from build123d import *

# Parameters (mm, degrees)
SKETCH1_W           = 261.5
SKETCH1_H           = 125.5
SKETCH1_R           = 2.5
SKETCH1_R_2         = 1.59
SKETCH1_R_3         = 2.1
SKETCH1_R_4         = 11.75
SKETCH1_W_2         = 33
SKETCH1_H_2         = 90
BOSS_EXTRUDE1_DEPTH = 5
CUT_EXTRUDE1_DEPTH  = 10
FILLET1_R           = 10
FILLET2_R           = 10


with BuildPart() as part:
    # Sketch1 → Boss-Extrude1 (new body)
    with BuildSketch(Plane.XY):
        with Locations((130.75, -62.75)):
            Rectangle(SKETCH1_W, SKETCH1_H)
        with Locations((255, -37.25)):
            Circle(SKETCH1_R, mode=Mode.SUBTRACT)
        with Locations((255, -88.25)):
            Circle(SKETCH1_R, mode=Mode.SUBTRACT)
        with Locations((183.81, -47.125)):
            Circle(SKETCH1_R_2, mode=Mode.SUBTRACT)
        with Locations((164.76, -78.375)):
            Circle(SKETCH1_R_2, mode=Mode.SUBTRACT)
        with Locations((152.06, -78.375)):
            Circle(SKETCH1_R_2, mode=Mode.SUBTRACT)
        with Locations((43.875030639, -118.888854871)):
            Circle(SKETCH1_R_3, mode=Mode.SUBTRACT)
        with Locations((183.81, -78.375)):
            Circle(SKETCH1_R_2, mode=Mode.SUBTRACT)
        with Locations((145.71, -47.125)):
            Circle(SKETCH1_R_2, mode=Mode.SUBTRACT)
        with Locations((158.41, -47.125)):
            Circle(SKETCH1_R_2, mode=Mode.SUBTRACT)
        with Locations((171.11, -47.125)):
            Circle(SKETCH1_R_2, mode=Mode.SUBTRACT)
        with Locations((145.71, -78.375)):
            Circle(SKETCH1_R_2, mode=Mode.SUBTRACT)
        with Locations((158.41, -78.375)):
            Circle(SKETCH1_R_2, mode=Mode.SUBTRACT)
        with Locations((171.11, -78.375)):
            Circle(SKETCH1_R_2, mode=Mode.SUBTRACT)
        with Locations((84.04, -78.375)):
            Circle(SKETCH1_R_2, mode=Mode.SUBTRACT)
        with Locations((96.74, -78.375)):
            Circle(SKETCH1_R_2, mode=Mode.SUBTRACT)
        with Locations((109.44, -78.375)):
            Circle(SKETCH1_R_2, mode=Mode.SUBTRACT)
        with Locations((84.04, -47.125)):
            Circle(SKETCH1_R_2, mode=Mode.SUBTRACT)
        with Locations((96.74, -47.125)):
            Circle(SKETCH1_R_2, mode=Mode.SUBTRACT)
        with Locations((109.44, -47.125)):
            Circle(SKETCH1_R_2, mode=Mode.SUBTRACT)
        with Locations((90.39, -78.375)):
            Circle(SKETCH1_R_2, mode=Mode.SUBTRACT)
        with Locations((103.09, -78.375)):
            Circle(SKETCH1_R_2, mode=Mode.SUBTRACT)
        with Locations((115.79, -78.375)):
            Circle(SKETCH1_R_2, mode=Mode.SUBTRACT)
        with Locations((90.39, -47.125)):
            Circle(SKETCH1_R_2, mode=Mode.SUBTRACT)
        with Locations((103.09, -47.125)):
            Circle(SKETCH1_R_2, mode=Mode.SUBTRACT)
        with Locations((115.79, -47.125)):
            Circle(SKETCH1_R_2, mode=Mode.SUBTRACT)
        with Locations((77.69, -78.375)):
            Circle(SKETCH1_R_2, mode=Mode.SUBTRACT)
        with Locations((5.1, -106.71894941)):
            Circle(SKETCH1_R_3, mode=Mode.SUBTRACT)
        with Locations((24.315775518, -112.75)):
            Circle(SKETCH1_R_4, mode=Mode.SUBTRACT)
        with Locations((256.4, -106.71894941)):
            Circle(SKETCH1_R_3, mode=Mode.SUBTRACT)
        with Locations((77.69, -47.125)):
            Circle(SKETCH1_R_2, mode=Mode.SUBTRACT)
        with Locations((6.5, -88.25)):
            Circle(SKETCH1_R, mode=Mode.SUBTRACT)
        with Locations((6.5, -37.25)):
            Circle(SKETCH1_R, mode=Mode.SUBTRACT)
        with Locations((237.184224482, -112.75)):
            Circle(SKETCH1_R_4, mode=Mode.SUBTRACT)
        with Locations((217.624969361, -118.888854871)):
            Circle(SKETCH1_R_3, mode=Mode.SUBTRACT)
        with Locations((152.06, -47.125)):
            Circle(SKETCH1_R_2, mode=Mode.SUBTRACT)
        with Locations((164.76, -47.125)):
            Circle(SKETCH1_R_2, mode=Mode.SUBTRACT)
        with Locations((177.46, -47.125)):
            Circle(SKETCH1_R_2, mode=Mode.SUBTRACT)
        with Locations((177.46, -78.375)):
            Circle(SKETCH1_R_2, mode=Mode.SUBTRACT)
        with Locations((256.4, -18.78105059)):
            Circle(SKETCH1_R_3, mode=Mode.SUBTRACT)
        with Locations((237.184224482, -12.75)):
            Circle(SKETCH1_R_4, mode=Mode.SUBTRACT)
        with Locations((217.624969361, -6.611145129)):
            Circle(SKETCH1_R_3, mode=Mode.SUBTRACT)
        with Locations((5.1, -18.78105059)):
            Circle(SKETCH1_R_3, mode=Mode.SUBTRACT)
        with Locations((43.875030639, -6.611145129)):
            Circle(SKETCH1_R_3, mode=Mode.SUBTRACT)
        with Locations((24.315775518, -12.75)):
            Circle(SKETCH1_R_4, mode=Mode.SUBTRACT)
        with Locations((206.31, -62.75)):
            Rectangle(SKETCH1_W_2, SKETCH1_H_2, mode=Mode.SUBTRACT)
        with Locations((55.19, -62.75)):
            Rectangle(SKETCH1_W_2, SKETCH1_H_2, mode=Mode.SUBTRACT)
    extrude(amount=BOSS_EXTRUDE1_DEPTH)

    # Sketch19 → Cut-Extrude1 (cut)
    with BuildSketch(Plane.XY.offset(5)):
        with BuildLine():
            Line((2.554773747, -112.220106382), (21.626568954, -125.5))
            Line((21.626568954, -125.5), (0, -125.5))
            Line((0, -125.5), (0, -108.394901529))
            ThreePointArc((0, -108.394901529), (0.915789995, -110.549006894), (2.554773747, -112.220106382))
        make_face()
        with BuildLine():
            Line((239.873431046, -125.5), (261.5, -125.5))
            Line((261.5, -125.5), (261.5, -108.394901529))
            ThreePointArc((261.5, -108.394901529), (260.584210005, -110.549006894), (258.945226253, -112.220106382))
            Line((258.945226253, -112.220106382), (239.873431046, -125.5))
        make_face()
        with BuildLine():
            Line((258.945226253, -13.279893618), (239.873431046, 0))
            Line((239.873431046, 0), (261.5, 0))
            Line((261.5, 0), (261.5, -17.105098471))
            ThreePointArc((261.5, -17.105098471), (260.584210005, -14.950993106), (258.945226253, -13.279893618))
        make_face()
        with BuildLine():
            Line((21.626568954, 0), (0, 0))
            Line((0, 0), (0, -17.105098471))
            ThreePointArc((0, -17.105098471), (0.915789995, -14.950993106), (2.554773747, -13.279893618))
            Line((2.554773747, -13.279893618), (21.626568954, 0))
        make_face()
        with BuildLine():
            ThreePointArc((68.905141109, -125.5), (130.75, -209.960536663), (192.594858891, -125.5))
            ThreePointArc((192.594858891, -125.5), (130.75, -80.215104564), (68.905141109, -125.5))
        make_face()
        with BuildLine():
            ThreePointArc((192.594858891, 0), (130.75, -45.284895436), (68.905141109, 0))
            ThreePointArc((68.905141109, 0), (130.75, 84.460536663), (192.594858891, 0))
        make_face()
    extrude(amount=-CUT_EXTRUDE1_DEPTH, mode=Mode.SUBTRACT)

    # Fillet1
    fillet1_edges = [part.edges().sort_by_distance(p)[0] for p in [
        (68.905141109, 0, 2.5),
        (192.594858891, 0, 2.5),
        (192.594858891, -125.5, 2.5),
        (68.905141109, -125.5, 2.5),
    ]]
    fillet(fillet1_edges, radius=FILLET1_R)

    # Fillet2
    fillet2_edges = [part.edges().sort_by_distance(p)[0] for p in [
        (239.873431046, 0, 2.5),
        (21.626568954, 0, 2.5),
        (21.626568954, -125.5, 2.5),
        (239.873431046, -125.5, 2.5),
    ]]
    fillet(fillet2_edges, radius=FILLET2_R)


solid = part.part
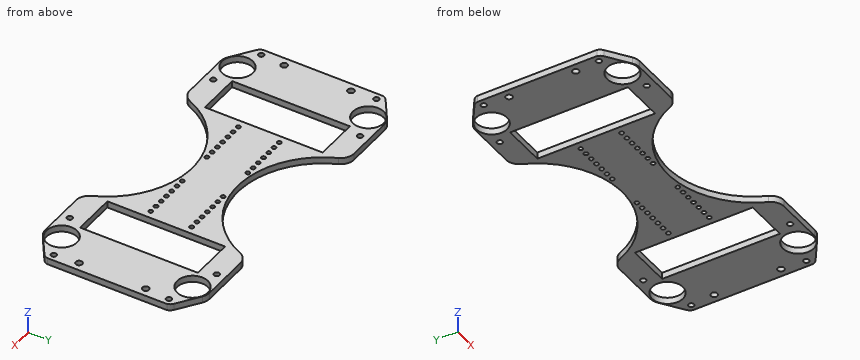
Work out the finished part from the listing and answer in its coordinate system (mm). Give positions to 0.01 mm unless a question says otherwise; leave off trailing zeros. Write each loop counter-clockwise with the first axis right and the second up, starting at its lowest first coordinate (ties: lowest second). Pieces come first, ordered by that corner, then holes. Notation, with made-up numbers: M 68,3 L 97,3 A25 ccw 97,22 Z; hole C 82.25,-11.5 d2. An arc over 180 degrees is marked long. Answer as CSV lines item,"result".
Q1. A cutting plane is placed at A-A on x = 52. Write down the section's boundary in (y, z), plus the area to 4 significant figures.
A:
outline,"M -125.5,0 L -107.75,0 L -107.75,5 L -125.5,5 Z; M -17.75,0 L 0,0 L 0,5 L -17.75,5 Z"
area,"177.5 mm²"
Q2. Find the intervals of material crossed by probe 1 along X at (y, z) = (-61, 3.3); probe 2 along Y at (x, z) = (77.69, 1.9) (3 decimals); probe 3 along Y at (x, z) = (246, 0.3), in increasing order. Write a range as [from, to].
A:
probe 1,"x = [0, 38.69], [71.69, 189.81], [222.81, 261.5]"
probe 2,"y = [-107.763, -79.965], [-76.785, -48.715], [-45.535, -17.737]"
probe 3,"y = [-121.23, -120.52], [-104.98, -20.52], [-4.98, -4.27]"
Q3. A cutting plane is placed at B-B on z = 1.85. Count the separate pieces of the cut face and the enclosed holes in it, plus the area to 3 significant figures.
A:
separate pieces,"1"
enclosed holes,"46"
area,"15,800 mm²"
Q4. Given P1, Ø3, axis at x = 171.11, y = -47.125, coming from the -Z side; P2, Ø1.5, axis at x = 157, z = 3.5, coming from the -Y side, each flat-ended and moving along its own axis, determine where each tip first touches the part or whether it passes through.
A:
P1,"passes through"
P2,"stops at y = -86.1"
